Read the model definition and answer for the solid it produces. Units are mm, in the model's axes. A direction names the side the tool comes from. Give positions to 0.01 mm unless a question says otherwise; leave off trailing zeros. Order: outer loops, then holes, each group sorted by start corner. A loop starts at its lowest first (then second) coordinate and runs counter-clockwise, first axis right, second up.
Item 1: Which of the six approach directions +Z, -Z, +X, -X, +Y, -Y give full straight-line access (tool end or side, diameter ignored) to faces 1 (the face through (0, -1, 2)), 2 (the face through (1.802, 3.958, 5.723)), 3 (the face through (3, -1, 0))?
Item 2: A cutting plane is placed at B-B (y = 4.25). Write down the section's boundary in (x, z).
Item 3: A cutting plane is placed at C-C (y = 8.75). Write down the section's boundary in (x, z).
Item 4: Find the intervals of material crossed by line 1 along X through (y, z) = (-0.25, 0.75); line 2 along Y through (x, z) = (-5.75, 5.5); line 3 along Y through (x, z) = (0.5, -3.75), in increasing order.
Item 5: A cutting plane is placed at D-D (y = 7.25). Write down the section's boundary in (x, z).
Item 6: A cutting plane is placed at A-A (z = 0). Write down the section's boundary in (x, y), plus the area to 3 significant figures.
Item 7: Given pin 1 Ø2 at (y, z) = (-0.5, 0) entering from +X; pin 2 Ø0.6 at (y, z) = (-1, -0.5) entering from -X; pin 3 Ø6 at (x, y) = (2, 7.5) entering from -Z; pin 4 Ø3 at (x, z) = (0, 0) entering from -Y, each flat-ended and moving along its own axis, determine where each tip first touches the part or whether it passes through.
from build123d import *

# Parameters (mm, degrees)
CROQUIS1_W              = 14
CROQUIS1_H              = 14
SALIENTE_EXTRUIR1_DEPTH = 1
CROQUIS2_W              = 4
CROQUIS2_H              = 4
CORTAR_EXTRUIR1_DEPTH   = 1
CROQUIS3_W              = 6
CROQUIS3_H              = 6
SALIENTE_EXTRUIR3_DEPTH = 1
CROQUIS5_W              = 4
CROQUIS5_H              = 4
CORTAR_EXTRUIR3_DEPTH   = 1
CROQUIS6_R              = 6
SALIENTE_EXTRUIR4_DEPTH = 8
CROQUIS7_W              = 6
CROQUIS7_H              = 6
CORTAR_EXTRUIR4_DEPTH   = 2
CROQUIS8_W              = 14
CROQUIS8_H              = 14
SALIENTE_EXTRUIR5_DEPTH = 1
CROQUIS9_W              = 6
CROQUIS9_H              = 6
SALIENTE_EXTRUIR6_DEPTH = 2
CROQUIS10_W             = 4
CROQUIS10_H             = 4
CORTAR_EXTRUIR5_DEPTH   = 2
REDONDEO2_R             = 2
CORTAR_EXTRUIR6_DEPTH   = 0.5


with BuildPart() as part:
    # Croquis1 → Saliente-Extruir1 (new body)
    with BuildSketch(Plane(origin=(0, 0, 0), x_dir=(1, 0, 0), z_dir=(0, 1, 0))):
        Rectangle(CROQUIS1_W, CROQUIS1_H)
    extrude(amount=SALIENTE_EXTRUIR1_DEPTH)

    # Croquis2 → Cortar-Extruir1 (cut)
    with BuildSketch(Plane.XZ):
        Rectangle(CROQUIS2_W, CROQUIS2_H)
    extrude(amount=-CORTAR_EXTRUIR1_DEPTH, mode=Mode.SUBTRACT)

    # Croquis3 → Saliente-Extruir3 (add)
    with BuildSketch(Plane.XZ):
        Rectangle(CROQUIS3_W, CROQUIS3_H)
    extrude(amount=SALIENTE_EXTRUIR3_DEPTH)

    # Croquis5 → Cortar-Extruir3 (cut)
    with BuildSketch(Plane.XZ.offset(1)):
        Rectangle(CROQUIS5_W, CROQUIS5_H)
    extrude(amount=-CORTAR_EXTRUIR3_DEPTH, mode=Mode.SUBTRACT)

    # Croquis6 → Saliente-Extruir4 (add)
    with BuildSketch(Plane(origin=(0, 1, 0), x_dir=(1, 0, 0), z_dir=(0, 1, 0))):
        with Locations(Location((0, 0, 0), (0, 0, 270))):
            Circle(CROQUIS6_R)
    extrude(amount=SALIENTE_EXTRUIR4_DEPTH)

    # Croquis7 → Cortar-Extruir4 (cut)
    with BuildSketch(Plane.XZ.offset(1)):
        Rectangle(CROQUIS7_W, CROQUIS7_H)
    extrude(amount=-CORTAR_EXTRUIR4_DEPTH, mode=Mode.SUBTRACT)

    # Croquis8 → Saliente-Extruir5 (add)
    with BuildSketch(Plane.XZ):
        Rectangle(CROQUIS8_W, CROQUIS8_H)
    extrude(amount=-SALIENTE_EXTRUIR5_DEPTH)

    # Croquis9 → Saliente-Extruir6 (add)
    with BuildSketch(Plane.XZ):
        Rectangle(CROQUIS9_W, CROQUIS9_H)
    extrude(amount=SALIENTE_EXTRUIR6_DEPTH)

    # Croquis10 → Cortar-Extruir5 (cut)
    with BuildSketch(Plane.XZ.offset(2)):
        Rectangle(CROQUIS10_W, CROQUIS10_H)
    extrude(amount=-CORTAR_EXTRUIR5_DEPTH, mode=Mode.SUBTRACT)

    # Redondeo2
    redondeo2_edges = [part.edges().sort_by_distance(p)[0] for p in [
        (0, 9, -6),
    ]]
    fillet(redondeo2_edges, radius=REDONDEO2_R)

    # Croquis11 → Cortar-Extruir6 (cut)
    with BuildSketch(Plane(origin=(0, 9, 0), x_dir=(1, 0, 0), z_dir=(0, 1, 0))):
        Polygon((0, 3), (-2.598076211, -1.5), (2.598076211, -1.5), align=None)
    extrude(amount=-CORTAR_EXTRUIR6_DEPTH, mode=Mode.SUBTRACT)


solid = part.part
Response values:
1. face 1: -Y
1. face 2: +Y
1. face 3: +Z, -Z, +X, -Y
2. outline: circle Ø12 at (0, 0)
3. outline: circle Ø9.94 at (0, 0); hole (-2.6, 1.5) - (0, -3) - (2.6, 1.5) - close
4. line 1: x = -3 to -2, 2 to 3
4. line 2: y = 0 to 1
4. line 3: y = 0 to 9
5. outline: circle Ø11.97 at (0, 0)
6. outline: (-7, 0) - (-3, 0) - (-3, -2) - (-2, -2) - (-2, 0) - (2, 0) - (2, -2) - (3, -2) - (3, 0) - (7, 0) - (7, 1) - (6, 1) - (6, 7) arc R2 ccw to (4, 9) - (1.73, 9) - (1.73, 8.5) - (-1.73, 8.5) - (-1.73, 9) - (-4, 9) arc R2 ccw to (-6, 7) - (-6, 1) - (-7, 1) - close
6. area: 111 mm2
7. pin 1: stops at x = 7
7. pin 2: stops at x = -3
7. pin 3: stops at z = -6
7. pin 4: stops at y = 0
